```python
from build123d import *

# Parameters (mm, degrees)
SKETCH1_W           = 75
SKETCH1_H           = 235.4
BOSS_EXTRUDE1_DEPTH = 5.7
SKETCH2_W           = 10
SKETCH2_H           = 5.7
CUT_EXTRUDE1_DEPTH  = 5.7
CUT_EXTRUDE2_DEPTH  = 5.7
CUT_EXTRUDE3_START  = -3.7
SKETCH4_R           = 1.5
CUT_EXTRUDE3_DEPTH  = 2


with BuildPart() as part:
    # Sketch1 → Boss-Extrude1 (new body)
    with BuildSketch(Plane.XY):
        with Locations((37.5, 117.7)):
            Rectangle(SKETCH1_W, SKETCH1_H)
    extrude(amount=BOSS_EXTRUDE1_DEPTH)

    # Sketch2 → Cut-Extrude1 (cut)
    with BuildSketch(Plane(origin=(0, 0, 0), x_dir=(-1, 0, 0), z_dir=(0, 0, -1))):
        with Locations((-70, 2.85)):
            Rectangle(SKETCH2_W, SKETCH2_H)
        with Locations((-5, 2.85)):
            Rectangle(SKETCH2_W, SKETCH2_H)
        with Locations((-5, 232.55)):
            Rectangle(SKETCH2_W, SKETCH2_H)
        with Locations((-70, 232.55)):
            Rectangle(SKETCH2_W, SKETCH2_H)
    extrude(amount=-CUT_EXTRUDE1_DEPTH, mode=Mode.SUBTRACT)

    # Sketch3 → Cut-Extrude2 (cut)
    with BuildSketch(Plane.XY.offset(5.7)):
        Polygon((57, 185), (55.55777949, 185), (17, 127.163330765), (17, 125), (18.44222051, 125), (57, 182.836669235), align=None)
        Polygon((52.67777949, 185), (49.79777949, 185), (17, 135.803330765), (17, 131.483330765), align=None)
        Polygon((46.91777949, 185), (44.03777949, 185), (17, 144.443330765), (17, 140.123330765), align=None)
        Polygon((41.15777949, 185), (38.27777949, 185), (17, 153.083330765), (17, 148.763330765), align=None)
        Polygon((35.39777949, 185), (32.51777949, 185), (17, 161.723330765), (17, 157.403330765), align=None)
        Polygon((29.63777949, 185), (26.75777949, 185), (17, 170.363330765), (17, 166.043330765), align=None)
        Polygon((23.87777949, 185), (20.99777949, 185), (17, 179.003330765), (17, 174.683330765), align=None)
        Polygon((57, 174.196669235), (57, 178.516669235), (21.32222051, 125), (24.20222051, 125), align=None)
        Polygon((57, 165.556669235), (57, 169.876669235), (27.08222051, 125), (29.96222051, 125), align=None)
        Polygon((57, 156.916669235), (57, 161.236669235), (32.84222051, 125), (35.72222051, 125), align=None)
        Polygon((57, 148.276669235), (57, 152.596669235), (38.60222051, 125), (41.48222051, 125), align=None)
        Polygon((57, 139.636669235), (57, 143.956669235), (44.36222051, 125), (47.24222051, 125), align=None)
        Polygon((57, 130.996669235), (57, 135.316669235), (50.12222051, 125), (53.00222051, 125), align=None)
    extrude(amount=-CUT_EXTRUDE2_DEPTH, mode=Mode.SUBTRACT)

    # Sketch4 → Cut-Extrude3 (cut)
    with BuildSketch(Plane.XY.offset(5.7).offset(CUT_EXTRUDE3_START)):
        with Locations((64.3, 20.7)):
            Circle(SKETCH4_R)
        with Locations((29.3, 20.7)):
            Circle(SKETCH4_R)
        with Locations((64.3, 214.7)):
            Circle(SKETCH4_R)
        with Locations((29.3, 214.7)):
            Circle(SKETCH4_R)
    extrude(amount=-CUT_EXTRUDE3_DEPTH, mode=Mode.SUBTRACT)


solid = part.part
```
Verification items for the finished model (mm, model axes). A direction names the side the tool comes from. Coordinates: 2 decimals unless noted, no trailing zeros. Loops run counter-clockwise (first coordinate to the right, second up) from the corner with the lowest first, then second, coordinate; pieces in that order, holes last. Notation, with made-up numbers: (-39, -17) -> (18, -17) arc R31 ccw to (18, 22) -> close; hole circle Ø5 at (63, -36). An arc over 180 degrees is marked (long way). Answer in a Markdown table with one row per item. Add a question column.
1. Depth check by flat-ended pin: P1, Ø1.5, axis at x = 29, y = 215, coming from the -Z side; P2, Ø1.4, axis at x = 28, z = 4, coming from the -Y side. Enter the tip coordinate at first touch or a pass-through.
2. Access from +Z, -Z, +X, -X, +Y, -Y to the whole of each face (thin tool, end or side, straight path). Record for faces 4 (the face through (70, 5.7, 3)), 5 (the face through (21.947, 177.784, 2.89)), 6 (the face through (10, 3, 3)), 7 (the face through (10, 233, 3)).
3. Material ranges on probe 1 along Y at (x, z) = (64.3, 1.55); probe 2 along X at (y, z) = (21, 0.25); probe 3 along Y at (x, z) = (70, 1.55), recorded low to high. Write a range as [from, to].
4. Section check A-A, the plane z = 4.4. Give the number of separate pieces and of enclosed holes in the cut face, then the cut area to 3 significant figures.
5. Section check B-B, the plane x = 7. Enter the section's corners in (y, z), then the cut area to 3 significant figures.
6. Draft check along Y on faces 1 (the face through (37, 119, 0)), 2 (the face through (20.39, 179.77, 2.89)), 3 (the face through (37, 235.4, 3)). Enter one of: +Y half, -Y half, draft (parallel to the pull), parting line (faces both ways), or undercut.
Derived:
| question | item | result |
|---|---|---|
| 1 | P1 | stops at z = 2 |
| 1 | P2 | stops at y = 0 |
| 2 | face 4 | +Z, -Z, +X, -Y |
| 2 | face 5 | +Z, -Z |
| 2 | face 6 | +Z, -Z, -X, -Y |
| 2 | face 7 | +Z, -Z, -X, +Y |
| 3 | probe 1 | y = [0, 19.2], [22.2, 213.2], [216.2, 235.4] |
| 3 | probe 2 | x = [0, 27.83], [30.77, 62.83], [65.77, 75] |
| 3 | probe 3 | y = [5.7, 229.7] |
| 4 | separate pieces | 1 |
| 4 | enclosed holes | 13 |
| 4 | area | 16,200 mm² |
| 5 | outline | (5.7, 0) -> (229.7, 0) -> (229.7, 5.7) -> (5.7, 5.7) -> close |
| 5 | area | 1,280 mm² |
| 6 | face 1 | draft |
| 6 | face 2 | undercut |
| 6 | face 3 | +Y half |
